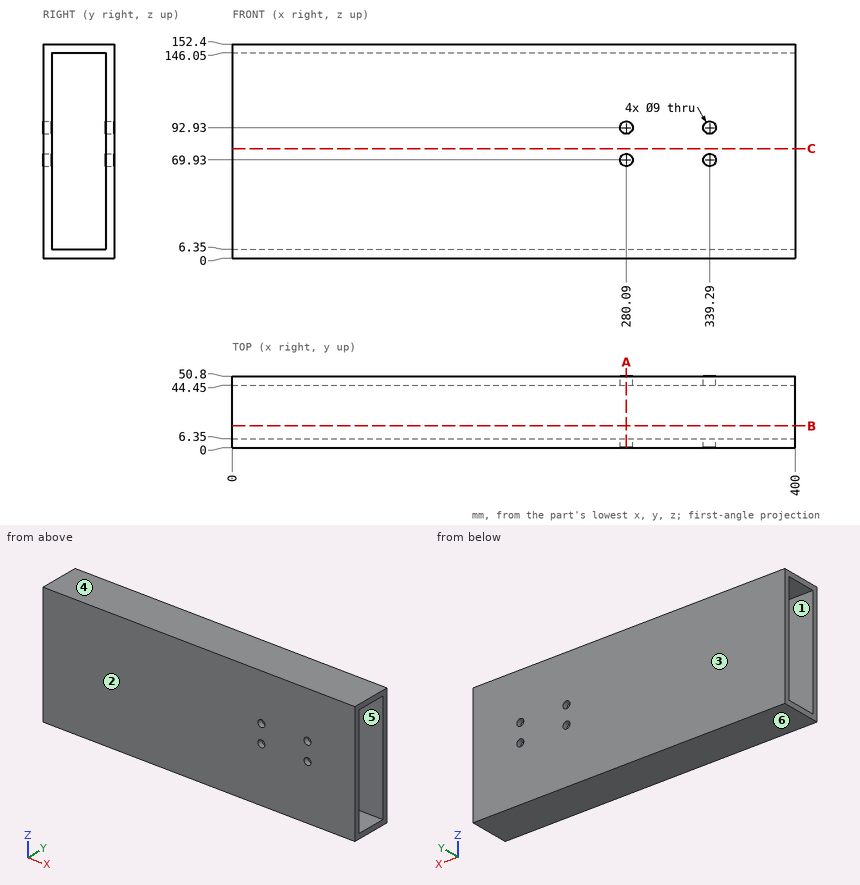
Verification items for this drawing (mm, ordinates from the low corner). A direction names the side the tool comes from. Coordinates: 2 decimals unless noted, no trailing zeros. Loops run counter-clockwise (first coordinate to the right, second up) from the corner with the lowest first, then second, coordinate; pieces in that order, holes last. Notation, with made-up numbers: (19.25, 79) -> (33.25, 79) arc R31 ccw to (33.25, 118) -> close; hole circle Ø9 at (33.5, 18). An arc over 180 degrees is marked (long way). Answer in a Markdown table with one row per item. Add a question column.
1. Material ranges on probe 1 along Z at (x, y) = (339, 3); probe 2 along X at (y, z) = (47.5, 92.93); probe 3 along Y at (x, z) = (215.5, 78.5), recorded low to high. Write a range as [from, to].
2. Section check B-B, the plane y = 15.5. Enter the section's corners in (x, z).
3. Access from +Z, -Z, +X, -X, +Y, -Y to the whole of each face (thin tool, end or side, straight path). Record for the marked faces 1 and 2.
4. Depth check by flat-ended pin: P1, Ø5.5, axis at x = 339.29, z = 69.93, coming from the +Y side. Enter the tip coordinate at first touch or a pass-through.
5. Section check C-C, the plane z = 78. Enter the section's corners in (x, y).
6. Section check A-A, the plane x = 280.09. Enter the section's corners in (y, z).
7. Draft check along Z on the marked faces 3, 4, 5 and 6. Enter one of: +Z half, -Z half, draft (parallel to the pull), parting line (faces both ways), or undercut.
Derived:
| question | item | result |
|---|---|---|
| 1 | probe 1 | z = [0, 65.44], [74.42, 88.44], [97.42, 152.4] |
| 1 | probe 2 | x = [0, 275.59], [284.59, 334.79], [343.79, 400] |
| 1 | probe 3 | y = [0, 6.35], [44.45, 50.8] |
| 2 | outline | (0, 0) -> (400, 0) -> (400, 6.35) -> (0, 6.35) -> close; (0, 146.05) -> (400, 146.05) -> (400, 152.4) -> (0, 152.4) -> close |
| 3 | face 1 | +X, -X |
| 3 | face 2 | +Z, -Z, +X, -X, -Y |
| 4 | P1 | passes through |
| 5 | outline | (0, 0) -> (400, 0) -> (400, 6.35) -> (0, 6.35) -> close; (0, 44.45) -> (400, 44.45) -> (400, 50.8) -> (0, 50.8) -> close |
| 6 | outline | (0, 0) -> (50.8, 0) -> (50.8, 65.43) -> (44.45, 65.43) -> (44.45, 6.35) -> (6.35, 6.35) -> (6.35, 65.43) -> (0, 65.43) -> close; (0, 74.43) -> (6.35, 74.43) -> (6.35, 88.43) -> (0, 88.43) -> close; (0, 97.43) -> (6.35, 97.43) -> (6.35, 146.05) -> (44.45, 146.05) -> (44.45, 97.43) -> (50.8, 97.43) -> (50.8, 152.4) -> (0, 152.4) -> close; (44.45, 74.43) -> (50.8, 74.43) -> (50.8, 88.43) -> (44.45, 88.43) -> close |
| 7 | face 3 | draft |
| 7 | face 4 | +Z half |
| 7 | face 5 | undercut |
| 7 | face 6 | -Z half |
